Geometry: see drawing. Coordinates: mm, zero at the bounding-box minimum. Give positions to 0.01 mm unless a question says otherwise; leave off trailing zeros. Write each loop counter-clockwise with the first axis right and the second up, starting at its lowest first coordinate (ties: lowest second). Pieces come first, ordered by that corner, then holes. Notation, with made-up numbers: M -14.75,-28.5 L 29.25,-28.5 A19 cw 29.25,-22.5 Z; hole C 41,63.5 d6. An arc over 180 degrees is marked long. Use a Markdown table: item, result. Add a question column.
1) Line query: line 1 (X direction, y = 0.65, z = 45.5); line 2 (X direction, y = 0.95, z = 3.5); line 3 (X direction, y = 0.45, z = 50.83). Output: solid intervals per line, ascending.
2) Section C-C on x = 66.1. Return the cut outline in (y, z).
3) Section A-A on y = 0.55. Return the cut outline in (x, z), then the cut area to 3 significant figures.
4) Section D-D on x = 90.2. Return the cut outline in (y, z), then the cut area to 3 significant figures.
5) Section B-B on z = 45.73. Return the cut outline in (x, y).
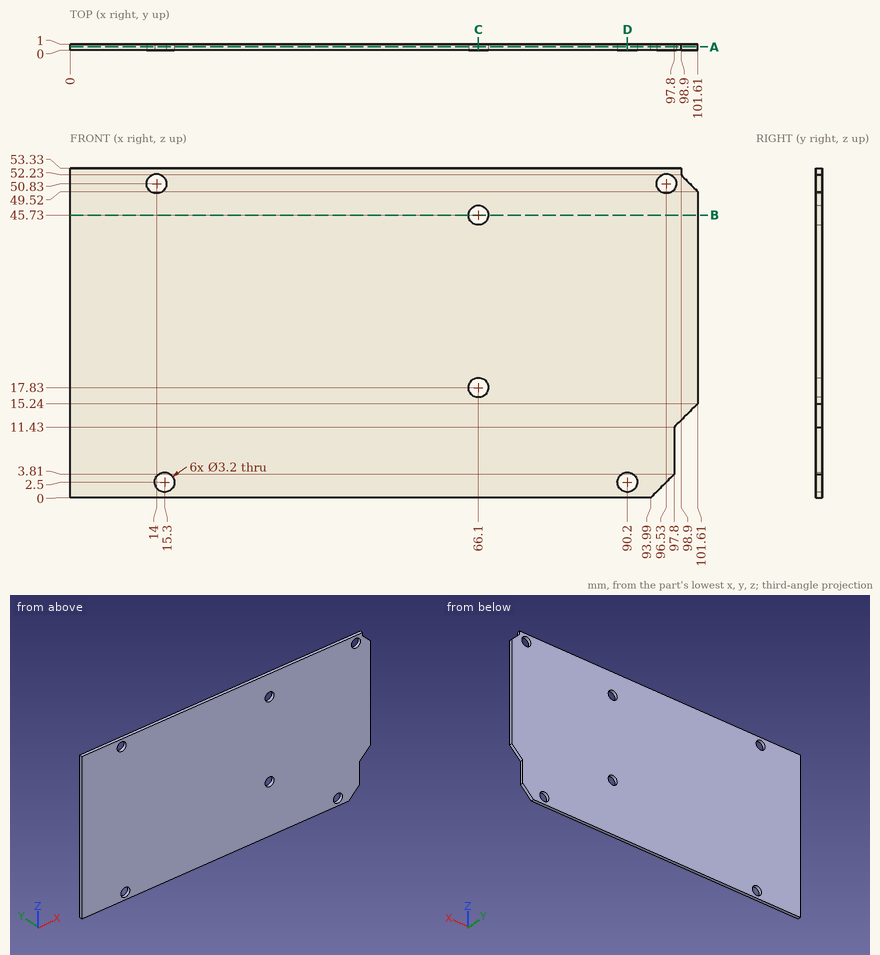
Found:
| question | item | result |
|---|---|---|
| 1 | line 1 | 0 to 64.52, 67.68 to 101.61 |
| 1 | line 2 | 0 to 14.05, 16.55 to 88.95, 91.45 to 97.49 |
| 1 | line 3 | 0 to 12.4, 15.6 to 94.93, 98.13 to 100.3 |
| 2 | outline | M 0,0 L 1,0 L 1,16.23 L 0,16.23 Z; M 0,19.43 L 1,19.43 L 1,44.13 L 0,44.13 Z; M 0,47.33 L 1,47.33 L 1,53.33 L 0,53.33 Z |
| 3 | outline | M 0,0 L 93.99,0 L 97.8,3.81 L 97.8,11.43 L 101.61,15.24 L 101.61,49.52 L 98.9,52.23 L 98.9,53.33 L 0,53.33 Z; hole C 14,50.83 d3.2; hole C 15.3,2.5 d3.2; hole C 66.1,17.83 d3.2; hole C 66.1,45.73 d3.2; hole C 90.2,2.5 d3.2; hole C 96.53,50.83 d3.2 |
| 3 | area | 5,310 mm² |
| 4 | outline | M 0,0 L 1,0 L 1,0.9 L 0,0.9 Z; M 0,4.1 L 1,4.1 L 1,53.33 L 0,53.33 Z |
| 4 | area | 50.1 mm² |
| 5 | outline | M 0,0 L 64.5,0 L 64.5,1 L 0,1 Z; M 67.7,0 L 101.61,0 L 101.61,1 L 67.7,1 Z |
